```python
from build123d import *

# Parameters (mm, degrees)
SKETCH1_W           = 36.83
SKETCH1_H           = 36.83
SKETCH1_W_2         = 28.702
SKETCH1_H_2         = 28.702
BOSS_EXTRUDE1_DEPTH = 50.8
FILLET1_R           = 2.54
SKETCH3_R           = 16.764
CUT_EXTRUDE2_DEPTH  = 66.39266874
CUT_EXTRUDE3_DEPTH  = 66.392668903
BOSS_EXTRUDE2_START = -127
SKETCH5_R           = 16.764
SKETCH5_R_2         = 14.605
BOSS_EXTRUDE2_DEPTH = 127


with BuildPart() as part:
    # Sketch1 → Boss-Extrude1 (new, symmetric)
    with BuildSketch(Plane(origin=(0, 0, 0), x_dir=(0, 0, -1), z_dir=(1, 0, 0))):
        Rectangle(SKETCH1_W, SKETCH1_H)
        Rectangle(SKETCH1_W_2, SKETCH1_H_2, mode=Mode.SUBTRACT)
    extrude(amount=BOSS_EXTRUDE1_DEPTH, both=True)

    # Fillet1
    fillet1_edges = [part.edges().sort_by_distance(p)[0] for p in [
        (0, -14.351, -14.351),
        (0, 14.351, -14.351),
        (0, 14.351, 14.351),
        (0, -14.351, 14.351),
        (0, 18.415, 18.415),
        (0, 18.415, -18.415),
        (0, -18.415, -18.415),
        (0, -18.415, 18.415),
    ]]
    fillet(fillet1_edges, radius=FILLET1_R)

    # Sketch3 → Cut-Extrude2 (cut, through all)
    with BuildSketch(Plane(origin=(0, 18.415, 0), x_dir=(1, 0, 0), z_dir=(0, 1, 0))):
        with Locations(Location((0, 0, 0), (0, 0, 251.257054082))):
            Circle(SKETCH3_R)
    extrude(amount=-CUT_EXTRUDE2_DEPTH, mode=Mode.SUBTRACT)

    # Sketch4 → Cut-Extrude3 (cut, through all)
    with BuildSketch(Plane(origin=(0, 18.415, 0), x_dir=(1, 0, 0), z_dir=(0, 1, 0))):
        with BuildLine():
            Line((-45.979437524, 18.415), (-50.8, 18.415))
            Line((-50.8, 18.415), (-50.8, -18.415))
            Line((-50.8, -18.415), (-45.979437524, -18.415))
            ThreePointArc((-45.979437524, -18.415), (-49.53, 0), (-45.979437524, 18.415))
        make_face()
        with BuildLine():
            Line((50.8, 15.875), (46.917004114, 15.875))
            ThreePointArc((46.917004114, 15.875), (48.872385422, 8.044305012), (49.53, 0))
            ThreePointArc((49.53, 0), (48.872385422, -8.044305012), (46.917004114, -15.875))
            Line((46.917004114, -15.875), (50.8, -15.875))
            Line((50.8, -15.875), (50.8, 15.875))
        make_face()
        with BuildLine():
            Line((50.8, 18.415), (45.979437524, 18.415))
            ThreePointArc((45.979437524, 18.415), (46.465579919, 17.151407603), (46.917004114, 15.875))
            Line((46.917004114, 15.875), (50.8, 15.875))
            Line((50.8, 15.875), (50.8, 18.415))
        make_face()
        with BuildLine():
            ThreePointArc((46.917004114, -15.875), (46.465579919, -17.151407603), (45.979437524, -18.415))
            Line((45.979437524, -18.415), (50.8, -18.415))
            Line((50.8, -18.415), (50.8, -15.875))
            Line((50.8, -15.875), (46.917004114, -15.875))
        make_face()
    extrude(amount=-CUT_EXTRUDE3_DEPTH, mode=Mode.SUBTRACT)

    # Sketch5 → Boss-Extrude2 (add)
    with BuildSketch(Plane.XZ.offset(18.415).offset(BOSS_EXTRUDE2_START)):
        with Locations(Location((0, 0, 0), (0, 0, 270))):
            Circle(SKETCH5_R)
        with Locations(Location((0, 0, 0), (0, 0, 270))):
            Circle(SKETCH5_R_2, mode=Mode.SUBTRACT)
    extrude(amount=BOSS_EXTRUDE2_DEPTH)


solid = part.part
```
The listing builds one solid part. Answer for the finished solid, in the listing's coordinates (mm). A direction names the side the tool comes from. Round coordinates to 2 decimals unless told otherwise and drop trailing zeros. Loops run counter-clockwise (first coordinate to the right, second up) from the corner with the lowest first, then second, coordinate; pieces in that order, holes last.
1) A cutting plane is placed at B-B on y = 4. Determine the outline of the cut face in (x, z) (3 decimals), plus the area to 3 significant figures.
Outcome:
outline: (-47.405, -14.351) arc R49.53 ccw to (-45.979, -18.415) - (45.979, -18.415) arc R49.53 ccw to (46.917, -15.875) arc R49.53 ccw to (47.405, -14.351) - (8.665, -14.351) arc R16.764 ccw to (8.665, 14.351) - (47.405, 14.351) arc R49.53 ccw to (46.917, 15.875) arc R49.53 ccw to (45.979, 18.415) - (-45.979, 18.415) arc R49.53 ccw to (-47.405, 14.351) - (-8.665, 14.351) arc R16.764 ccw to (-8.665, -14.351) - close; hole circle Ø29.21 at (0, 0)
area: 916 mm2
2) Consider line 1 (Y direction, x = -44, z = -9) (3 decimals); line 2 (X direction, y = 92, z = 0.5). Determine where each line is inside the solid, lowest interval first.
Outcome:
line 1: y = -18.415 to -14.351, 14.351 to 18.415
line 2: x = -16.76 to -14.6, 14.6 to 16.76
3) A cutting plane is placed at A-A on x = 0. Determine the outline of the cut face in (y, z) (3 decimals).
Outcome:
outline: (-18.415, -16.764) - (-18.254, -16.764) arc R2.54 ccw to (-15.875, -18.415) - (15.875, -18.415) arc R2.54 ccw to (18.254, -16.764) - (108.585, -16.764) - (108.585, -14.605) - (-18.415, -14.605) - close; (-18.415, 14.605) - (108.585, 14.605) - (108.585, 16.764) - (18.254, 16.764) arc R2.54 ccw to (15.875, 18.415) - (-15.875, 18.415) arc R2.54 ccw to (-18.254, 16.764) - (-18.415, 16.764) - close
4) For a pull along Z with two mould halves and no side action, classify faces 4 (the face through (-0.66, 17.65, -17.69)), 5 (the face through (-10.201, 64.052, 13.303)), 6 (the face through (28, 0, -14.351)), 7 (the face through (-28.107, -13.587, 13.627)) as released by +Z, released by -Z, zero draft, split by the parting line, or undercut.
Outcome:
face 4: released by -Z
face 5: split by the parting line
face 6: undercut
face 7: undercut
5) For faces 1 (the face through (-28.659, 13.627, -13.587)), 2 (the face through (1, 0, 18.415)), 3 (the face through (31, 14.351, 0)), determine the directions among +Z, -Z, +X, -X, +Y, -Y from which every point of the face is accessible in a straight line to the end or side of a thin tool.
Outcome:
face 1: -X
face 2: +Z, +X, -X, +Y, -Y
face 3: +X
6) Given P1, Ø16, axis at x = 30.5, z = 1.5, coming from the +Y side (3 decimals); P2, Ø1.5, axis at x = -2.5, y = 88, coming from the +Z side; P3, Ø12, axis at x = -21, y = 60.5, coming from the -Z side, each flat-ended and moving along its own axis, determine where each tip first touches the part or whether it passes through.
Outcome:
P1: stops at y = 18.415
P2: stops at z = 16.67
P3: stops at z = -7.49
7) A cutting plane is placed at C-C on z = 10. Determine the outline of the cut face in (x, y) (3 decimals), plus the area to 3 significant figures.
Outcome:
outline: (-48.51, -18.415) - (-10.645, -18.415) - (-10.645, 108.585) - (-13.455, 108.585) - (-13.455, 18.415) - (-48.51, 18.415) - (-48.51, 14.351) - (-13.455, 14.351) - (-13.455, -14.351) - (-48.51, -14.351) - close; (10.645, -18.415) - (48.51, -18.415) - (48.51, -14.351) - (13.455, -14.351) - (13.455, 14.351) - (48.51, 14.351) - (48.51, 18.415) - (13.455, 18.415) - (13.455, 108.585) - (10.645, 108.585) - close
area: 1,280 mm2
8) A cutting plane is placed at D-D on x = -37.5. Determine the outline of the cut face in (y, z) (3 decimals).
Outcome:
outline: (-18.415, -15.875) arc R2.54 ccw to (-15.875, -18.415) - (15.875, -18.415) arc R2.54 ccw to (18.415, -15.875) - (18.415, 15.875) arc R2.54 ccw to (15.875, 18.415) - (-15.875, 18.415) arc R2.54 ccw to (-18.415, 15.875) - close; hole (-14.351, -11.811) arc R2.54 ccw to (-11.811, -14.351) - (11.811, -14.351) arc R2.54 ccw to (14.351, -11.811) - (14.351, 11.811) arc R2.54 ccw to (11.811, 14.351) - (-11.811, 14.351) arc R2.54 ccw to (-14.351, 11.811) - close
